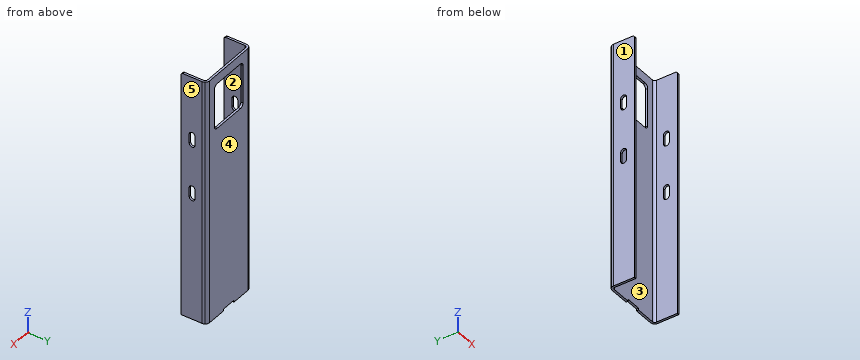
```python
from build123d import *

# Parameters (mm, degrees)
BOSS_EXTRUDE1_DEPTH        = 955
FLATTEN_BENDS1_OUTLINE_W   = 6
FLATTEN_BENDS1_OUTLINE_H   = 64
FLATTEN_BENDS1_DEPTH       = 955
FLATTEN_BENDS1_2_OUTLINE_W = 59.495264307
FLATTEN_BENDS1_2_OUTLINE_H = 6
FLATTEN_BENDS1_2_DEPTH     = 955
PROCESS_BENDS1_DEPTH       = 955
PROCESS_BENDS1_2_DEPTH     = 955
BOSS_EXTRUDE2_DEPTH        = 6
EDGE_FLANGE1_DEPTH         = 206.725155702
EDGE_FLANGE1_BEND_DEPTH    = 206.725155702
CUT_EXTRUDE1_DEPTH         = 15
CUT_EXTRUDE2_START         = -25.25
CUT_EXTRUDE2_DEPTH         = 25.25
SKETCH17_W                 = 20.5
SKETCH17_H                 = 7
CUT_EXTRUDE3_DEPTH         = 10
FILLET1_R                  = 10
SKETCH18_W                 = 41
SKETCH18_H                 = 5.25
CUT_EXTRUDE4_DEPTH         = 10
SKETCH19_W                 = 174
SKETCH19_H                 = 480
CUT_EXTRUDE5_DEPTH         = 1164.457508004
FILLET2_R                  = 5
CUT_EXTRUDE6_DEPTH         = 704.546245741


# Read off the part's stored shape, not the designer's step: Flatten-Bends1, Process-Bends1, Cut-Extrude2
# Sheet-metal steps are written as plain solids
with BuildPart() as part:
    # Sketch1 → Boss-Extrude1 (new body)
    with BuildSketch(Plane.XY):
        Polygon((-87, -70), (-87, 0), (87, 0), (87, -70), (81, -70), (81, -6), (-81, -6), (-81, -70), align=None)
    extrude(amount=BOSS_EXTRUDE1_DEPTH)

    # Flatten-Bends1 outline → Flatten-Bends1 (cut)
    with BuildSketch(Plane.XY):
        with Locations((-84, -38)):
            Rectangle(FLATTEN_BENDS1_OUTLINE_W, FLATTEN_BENDS1_OUTLINE_H)
        with Locations((84, -38)):
            Rectangle(FLATTEN_BENDS1_OUTLINE_W, FLATTEN_BENDS1_OUTLINE_H)
    extrude(amount=FLATTEN_BENDS1_DEPTH, mode=Mode.SUBTRACT)

    # Flatten-Bends1 2 outline → Flatten-Bends1 2 (add)
    with BuildSketch(Plane.XY):
        with Locations((-116.747632154, -3)):
            Rectangle(FLATTEN_BENDS1_2_OUTLINE_W, FLATTEN_BENDS1_2_OUTLINE_H)
        with Locations((116.747632154, -3)):
            Rectangle(FLATTEN_BENDS1_2_OUTLINE_W, FLATTEN_BENDS1_2_OUTLINE_H)
    extrude(amount=FLATTEN_BENDS1_2_DEPTH)

    # Process-Bends1 outline → Process-Bends1 (cut)
    with BuildSketch(Plane.XY):
        with BuildLine():
            ThreePointArc((74.8, 0), (80.849793384, -1.60566189), (85.307140429, -6))
            Line((85.307140429, -6), (146.495264307, -6))
            Line((146.495264307, -6), (146.495264307, 0))
            Line((146.495264307, 0), (74.8, 0))
        make_face()
        with BuildLine():
            Line((-146.495264307, -6), (-85.307140429, -6))
            ThreePointArc((-85.307140429, -6), (-80.849793384, -1.60566189), (-74.8, 0))
            Line((-74.8, 0), (-146.495264307, 0))
            Line((-146.495264307, 0), (-146.495264307, -6))
        make_face()
    extrude(amount=PROCESS_BENDS1_DEPTH, mode=Mode.SUBTRACT)

    # Process-Bends1 2 outline → Process-Bends1 2 (add)
    with BuildSketch(Plane.XY):
        with BuildLine():
            Line((81, -12.2), (81, -70))
            Line((81, -70), (87, -70))
            Line((87, -70), (87, -12.2))
            ThreePointArc((87, -12.2), (86.569178247, -8.986521607), (85.307140429, -6))
            Line((85.307140429, -6), (74.8, -6))
            ThreePointArc((74.8, -6), (79.184062043, -7.815937957), (81, -12.2))
        make_face()
        with BuildLine():
            Line((-87, -70), (-81, -70))
            Line((-81, -70), (-81, -12.2))
            ThreePointArc((-81, -12.2), (-79.184062043, -7.815937957), (-74.8, -6))
            Line((-74.8, -6), (-85.307140429, -6))
            ThreePointArc((-85.307140429, -6), (-86.569178247, -8.986521607), (-87, -12.2))
            Line((-87, -12.2), (-87, -70))
        make_face()
    extrude(amount=PROCESS_BENDS1_2_DEPTH)

    # Sketch8 → Boss-Extrude2 (add)
    with BuildSketch(Plane(origin=(0, 0, 0), x_dir=(1, 0, 0), z_dir=(0, 1, 0))):
        Polygon((-74.8, -955), (-22.5, -1155), (22.5, -1155), (74.8, -955), align=None)
    extrude(amount=-BOSS_EXTRUDE2_DEPTH)

    # Edge-Flange1 section (across the edge) → Edge-Flange1 (add)
    with BuildSketch(Plane(origin=(80.798302412, -6, 956.568556081), x_dir=(-0.9674681309145718, -3.491481338843133e-15, -0.25299291623416037), z_dir=(-0.25299291623416037, 0, 0.9674681309145718))):
        with BuildLine():
            Line((-6, 6.2), (-6, 64))
            Line((-6, 64), (0, 64))
            Line((0, 64), (0, 6.2))
            ThreePointArc((0, 6.2), (1.815937957, 1.815937957), (6.2, 0))
            Line((6.2, 0), (6.2, -6))
            ThreePointArc((6.2, -6), (-2.42670273, -2.42670273), (-6, 6.2))
        make_face()
    extrude(amount=EDGE_FLANGE1_DEPTH)

    # Edge-Flange1 section 2 (across the edge) → Edge-Flange1 bend (add)
    with BuildSketch(Plane(origin=(-28.498302412, -6, 1156.568556081), x_dir=(0.9674681309145718, -3.4914813388431337e-15, -0.25299291623416087), z_dir=(-0.25299291623416087, 0, -0.9674681309145718))):
        with BuildLine():
            Line((-6, 6.2), (-6, 64))
            Line((-6, 64), (0, 64))
            Line((0, 64), (0, 6.2))
            ThreePointArc((0, 6.2), (1.815937957, 1.815937957), (6.2, 0))
            Line((6.2, 0), (6.2, -6))
            ThreePointArc((6.2, -6), (-2.42670273, -2.42670273), (-6, 6.2))
        make_face()
    extrude(amount=EDGE_FLANGE1_BEND_DEPTH)

    # Sketch15 → Cut-Extrude1 (cut)
    with BuildSketch(Plane(origin=(0, 0, 0), x_dir=(1, 0, 0), z_dir=(0, 1, 0))):
        with BuildLine():
            Line((46, -652.45), (-46, -652.45))
            ThreePointArc((-46, -652.45), (-53.071067812, -649.521067812), (-56, -642.45))
            Line((-56, -642.45), (-56, -537.45))
            ThreePointArc((-56, -537.45), (-53.071067812, -530.378932188), (-46, -527.45))
            Line((-46, -527.45), (46, -527.45))
            ThreePointArc((46, -527.45), (53.071067812, -530.378932188), (56, -537.45))
            Line((56, -537.45), (56, -642.45))
            ThreePointArc((56, -642.45), (53.071067812, -649.521067812), (46, -652.45))
        make_face()
    extrude(amount=-CUT_EXTRUDE1_DEPTH, mode=Mode.SUBTRACT)

    # Cut-Extrude2 outline → Cut-Extrude2 (cut)
    with BuildSketch(Plane.XZ.offset(70).offset(CUT_EXTRUDE2_START)):
        Polygon((-53.676734498, 1084), (-47.871925712, 1082.482042503), (-45.644479827, 1091), (-51.449288612, 1092.517957497), align=None)
        Polygon((45.644479827, 1091), (47.871925713, 1082.482042503), (53.676734498, 1084), (51.449288612, 1092.517957497), align=None)
    extrude(amount=CUT_EXTRUDE2_DEPTH, mode=Mode.SUBTRACT)

    # Sketch17 → Cut-Extrude3 (cut)
    with BuildSketch(Plane.XZ.offset(6)):
        with Locations((0, 1087.5)):
            Rectangle(SKETCH17_W, SKETCH17_H)
    extrude(amount=-CUT_EXTRUDE3_DEPTH, mode=Mode.SUBTRACT)

    # Fillet1
    fillet1_edges = [part.edges().sort_by_distance(p)[0] for p in [
        (31.400706804, -70, 1157.327534829),
        (-31.400706804, -70, 1157.327534829),
    ]]
    fillet(fillet1_edges, radius=FILLET1_R)

    # Sketch18 → Cut-Extrude4 (cut)
    with BuildSketch(Plane(origin=(0, 0, 0), x_dir=(1, 0, 0), z_dir=(0, 1, 0))):
        with Locations((0, -2.625)):
            Rectangle(SKETCH18_W, SKETCH18_H)
    extrude(amount=-CUT_EXTRUDE4_DEPTH, mode=Mode.SUBTRACT)

    # Sketch19 → Cut-Extrude5 (cut, through all)
    with BuildSketch(Plane(origin=(0, 0, 0), x_dir=(1, 0, 0), z_dir=(0, 1, 0))):
        with Locations((0, -918.086513578)):
            Rectangle(SKETCH19_W, SKETCH19_H)
    extrude(amount=-CUT_EXTRUDE5_DEPTH, mode=Mode.SUBTRACT)

    # Fillet2
    fillet2_edges = [part.edges().sort_by_distance(p)[0] for p in [
        (84, -70, 678.086513578),
        (-84, -70, 678.086513578),
    ]]
    fillet(fillet2_edges, radius=FILLET2_R)

    # Sketch20 → Cut-Extrude6 (cut, through all)
    with BuildSketch(Plane.ZY.offset(87)):
        with BuildLine():
            Line((490.586513578, -32), (515.586513578, -32))
            ThreePointArc((515.586513578, -32), (523.586513578, -40), (515.586513578, -48))
            Line((515.586513578, -48), (490.586513578, -48))
            ThreePointArc((490.586513578, -48), (482.586513578, -40), (490.586513578, -32))
        make_face()
        with BuildLine():
            Line((365.586513578, -32), (340.586513578, -32))
            ThreePointArc((340.586513578, -32), (332.586513578, -40), (340.586513578, -48))
            Line((340.586513578, -48), (365.586513578, -48))
            ThreePointArc((365.586513578, -48), (373.586513578, -40), (365.586513578, -32))
        make_face()
    extrude(amount=-CUT_EXTRUDE6_DEPTH, mode=Mode.SUBTRACT)


solid = part.part
```
Read the model definition and answer for the solid it produces. Units are mm, in the model's axes. Face numbers are marked on the shaded views. A direction names the side the tool comes from. Coordinates: 2 decimals unless noted, no trailing zeros. Order: outer loops, then holes, each group sorted by start corner. A loop starts at its lowest first (then second) coordinate and runs counter-clockwise, first axis right, second up. Notation, with made-up numbers: (-21.5, 2.5) - (20.5, 2.5) arc R10 cw to (20.5, 10.5) - close; hole circle Ø10 at (-11.5, 48.5). An arc over 180 degrees is marked (long way). Answer as a JSON object with one key per item and string values. Group by question number.
Item 1: The mould has two halves that part along X. Classify the marked faces 3, 4 and 5: +X half, -X half, draft (parallel to the pull), parting line (faces both ways), or undercut.
Item 2: Section D-D (z = 109.5) is taken. Give the vertices of the cut face in (x, y), plus the area to 3 significant figures.
Item 3: Section C-C (y = -40) is taken. Give the vertices of the cut face in (x, z), plus the area to 3 significant figures.
Item 4: Flat-ended cylindrical pins translate along their axes: P1, Ø5, axis at x = 84, z = 506, coming from the +Y side; P2, Ø5, axis at y = -4, z = 605, coming from the +X side; P3, Ø3, axis at x = -38, y = -9, coming from the +Z side; P4, Ø6.5, axis at x = 6.5, y = -3.5, coming from the -Z side. Find the tip coordinate at first contact, or state that the pin passes through.
Item 5: Consider probe 1 along X at (y, z) = (-17, 380.5); probe 2 along Z at (x, y) = (10, -5.5); probe 3 along Y at (x, z) = (32.5, 269). Determine where each line is inside the solid, lowest interval first. Write a range as from..to.
Item 6: Section B-B (x = 29.5) is taken. Give the vertices of the cut face in (y, z).
Item 7: Section A-A (z = 565) is taken. Give the vertices of the cut face in (x, y).
Item 8: A tool of negligible diameter and unlimited length cuts with its end or side. For the marked faces 1 and 2, from which of +Z, -Z, +X, -X, +Y, -Y can it reach the whole face along a straight path? Write none if from no direction.
Results are:
{
 "1": {"face 3": "undercut", "face 4": "draft", "face 5": "+X half"},
 "2": {"outline": "(-87, -70) - (-81, -70) - (-81, -12.2) arc R6.2 cw to (-74.8, -6) - (74.8, -6) arc R6.2 cw to (81, -12.2) - (81, -70) - (87, -70) - (87, -12.2) arc R12.2 ccw to (74.8, 0) - (-74.8, 0) arc R12.2 ccw to (-87, -12.2) - close", "area": "1,760 mm^2"},
 "3": {"outline": "(-87, 0) - (-81, 0) - (-81, 332.59) - (-87, 332.59) - close; (-87, 373.59) - (-81, 373.59) - (-81, 482.59) - (-87, 482.59) - close; (-87, 523.59) - (-81, 523.59) - (-81, 678.09) - (-87, 678.09) - close; (81, 0) - (87, 0) - (87, 332.59) - (81, 332.59) - close; (81, 373.59) - (87, 373.59) - (87, 482.59) - (81, 482.59) - close; (81, 523.59) - (87, 523.59) - (87, 678.09) - (81, 678.09) - close", "area": "7,150 mm^2"},
 "4": {"P1": "stops at y = -2", "P2": "stops at x = 85.59", "P3": "passes through", "P4": "stops at z = 5.25"},
 "5": {"probe 1": "x = -87..-81, 81..87", "probe 2": "z = 5.25..527.45, 652.45..678.09", "probe 3": "y = -6..0"},
 "6": {"outline": "(-6, 0) - (0, 0) - (0, 527.45) - (-6, 527.45) - close; (-6, 652.45) - (0, 652.45) - (0, 678.09) - (-6, 678.09) - close"},
 "7": {"outline": "(-87, -70) - (-81, -70) - (-81, -12.2) arc R6.2 cw to (-74.8, -6) - (-56, -6) - (-56, 0) - (-74.8, 0) arc R12.2 ccw to (-87, -12.2) - close; (56, -6) - (74.8, -6) arc R6.2 cw to (81, -12.2) - (81, -70) - (87, -70) - (87, -12.2) arc R12.2 ccw to (74.8, 0) - (56, 0) - close"},
 "8": {"face 1": "+Z, -Z, -X, +Y, -Y", "face 2": "+Z, -Z, -Y"}
}
